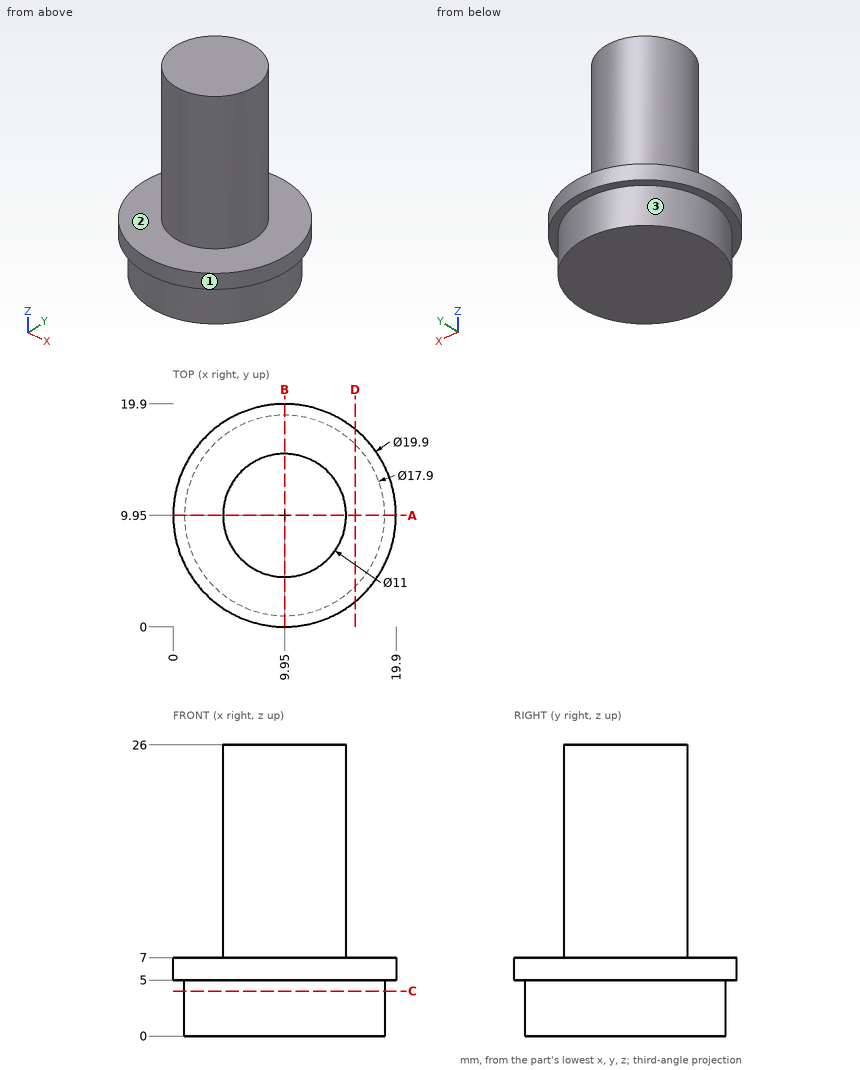
The drawing under review shows one solid part. Ordinate dimensions are in mm from its lowest x, y, z. A direction names the side the tool comes from. Round coordinates to 2 decimals unless told otherwise and drop trailing zeros. Order: outer loops, then holes, each group sorted by start corner. A loop starts at its lowest first (then second) coordinate and runs counter-clockwise, first axis right, second up. Notation, with made-up numbers: (-25, -20) - (-18, -20) arc R11 ccw to (-18, -14) - close; hole circle Ø3 at (43.5, 30.25). An arc over 180 degrees is marked (long way). Return JSON: item names as keys, results as strings.
Q1. Wall thickness on L1, parallel to Z at x = 9.75, y = 1.5; L2, parallel to Z at x = 2.5, y = 16; L3, parallel to X at y = 14.5, z = 11: over which ranges is each line inside the solid? List them lowest first. Write a range as [from, to].
Computed values:
{"L1": "z = [0, 7]", "L2": "z = [5, 7]", "L3": "x = [6.86, 13.04]"}
Q2. Consider section A-A on y = 9.95. Write out the cut boundary in (x, z), plus the area to 3 significant figures.
Computed values:
{"outline": "(0, 5) - (1, 5) - (1, 0) - (18.9, 0) - (18.9, 5) - (19.9, 5) - (19.9, 7) - (15.45, 7) - (15.45, 26) - (4.45, 26) - (4.45, 7) - (0, 7) - close", "area": "338 mm2"}
Q3. Consider section D-D on x = 16.25. Write out the cut boundary in (y, z).
Computed values:
{"outline": "(2.25, 5) - (3.59, 5) - (3.59, 0) - (16.31, 0) - (16.31, 5) - (17.65, 5) - (17.65, 7) - (2.25, 7) - close"}
Q4. Consider section C-C on z = 4. Write out the cut boundary in (x, y), plus the area to 3 significant figures.
Computed values:
{"outline": "circle Ø17.9 at (9.95, 9.95)", "area": "252 mm2"}
Q5. Machinability: for the marked faces 1, 2 and 3, which of the approach directions +Z, -Z, +X, -X, +Y, -Y give a long, thin tool a straight path to every point of the face, cutting with its end or side? Answer none if there is none.
Computed values:
{"face 1": "+Z, -Z", "face 2": "+Z", "face 3": "-Z"}
Q6. For pin 1 Ø1 at (x, z) = (15.5, 12.5) entering from +Y; pin 2 Ø3 at (x, z) = (4, 18) entering from -Y; pin 3 Ø3 at (x, z) = (9.5, 15) entering from -Y; pin 4 Ø1 at (x, y) = (3, 14.5) entering from -Z, all flat-tipped, find the tip position at first contact; note any pin that passes through.
Computed values:
{"pin 1": "stops at y = 12.13", "pin 2": "stops at y = 6.72", "pin 3": "stops at y = 4.45", "pin 4": "stops at z = 0"}
